The figure shows three views and two pictorial views of one solid part (mm, origin at its lowest corner). Answer the questions. A direction names the side the tool comes from. Round coordinates to 2 decimals unless told otherwise and drop trailing zeros. Order: outer loops, then holes, each group sorted by start corner. A loop starts at its lowest first (then second) coordinate and runs counter-clockwise, first axis right, second up. Notation, with made-up numbers: (53.25, 1) - (64.25, 1) arc R17 ccw to (64.25, 27) - close; hole circle Ø6 at (83, 49). An arc over 180 degrees is marked (long way). Use CSV: the item, a comma, the result in double quotes. Start each with the question number.
Item 1: Flat-ended cylindrical pins translate along their axes: P1, Ø4.5, axis at x = 7, y = 7, coming from the +Z side; P2, Ø1.5, axis at y = 5.5, z = 4, coming from the -X side; P3, Ø2, axis at y = 9, z = 14.5, coming from the +X side; P4, Ø1.5, axis at x = 8.5, z = 15, coming from the +Y side. Find the tip coordinate at first contact, or state that the pin passes through.
Item 2: Find section A-A, the plane y = 7. Give the vertices of the cut face in (x, z), plus the area to 4 significant figures.
Item 3: Determine the mould class of the marked faces 1, 2 and 3 for opening direction X: +X half, -X half, draft (parallel to the pull), parting line (faces both ways), or undercut.
Item 4: Find section D-D, the plane z = 21.5. Give the vertices of the cut face in (x, y).
Item 5: For the marked faces 4 and 5, determine the directions among +Z, -Z, +X, -X, +Y, -Y from which every point of the face is accessible in a straight line to the end or side of a thin tool.
Item 6: Straight lines are drawn through the part: line 1 along Y through (x, z) = (7, 7.25); line 2 along Y through (x, z) = (7, 22.25); line 3 along Z through (x, y) = (9.5, 5.75). For each, find the intervals that lie inside material, in ascending order. Write a range as [from, to].
Item 7: Find section C-C, the plane z = 2. Give the vertices of the cut face in (x, y), plus the area to 3 significant figures.
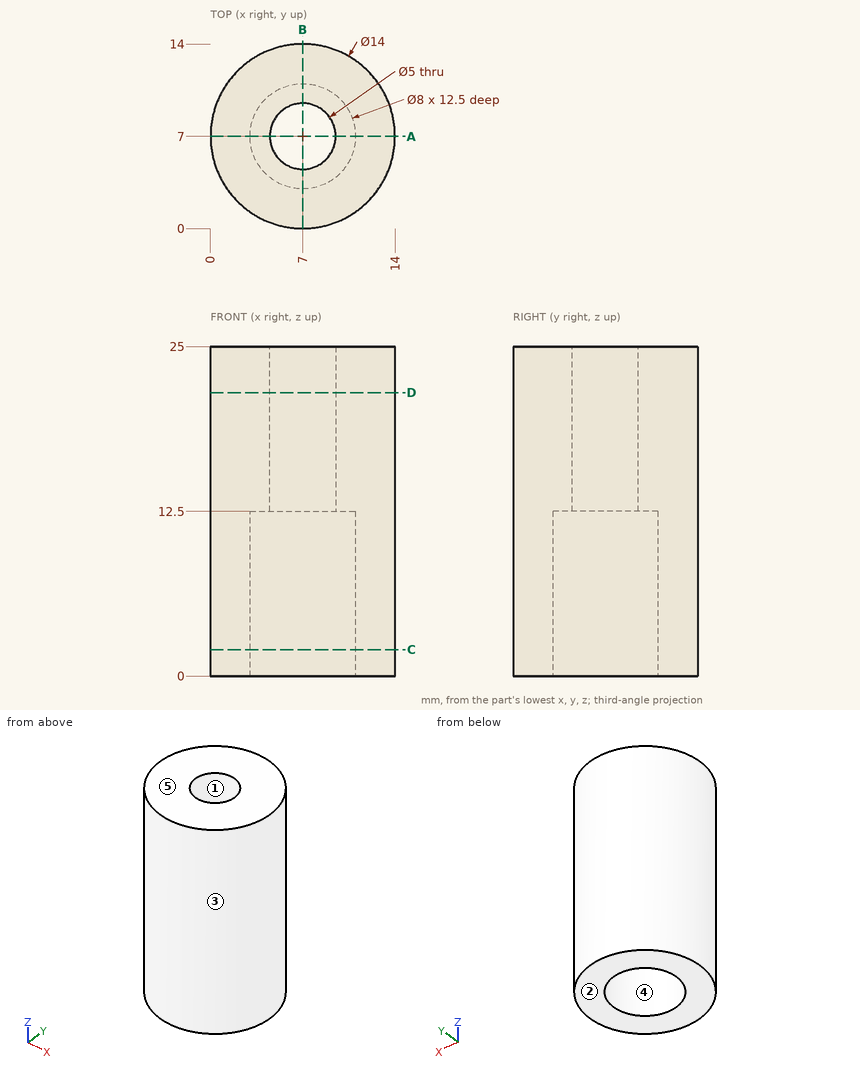
Worked out:
1,P1,"passes through"
1,P2,"stops at x = 0.04"
1,P3,"stops at x = 13.93"
1,P4,"stops at y = 13.96"
2,outline,"(0, 0) - (3, 0) - (3, 12.5) - (4.5, 12.5) - (4.5, 25) - (0, 25) - close; (9.5, 12.5) - (11, 12.5) - (11, 0) - (14, 0) - (14, 25) - (9.5, 25) - close"
2,area,"187.5 mm²"
3,face 1,"undercut"
3,face 2,"draft"
3,face 3,"parting line"
4,outline,"circle Ø14 at (7, 7); hole circle Ø5 at (7, 7)"
5,face 4,"-Z"
5,face 5,"+Z, +X, -X, +Y, -Y"
6,line 1,"y = [0, 3], [11, 14]"
6,line 2,"y = [0, 4.5], [9.5, 14]"
6,line 3,"z = [12.5, 25]"
7,outline,"circle Ø14 at (7, 7); hole circle Ø8 at (7, 7)"
7,area,"104 mm²"
